CAD build for the part. Positions are in the model's coordinates, mm. A direction names the side the tool comes from. Give positions to 0.01 mm unless a question says otherwise; leave off trailing zeros. Loops run counter-clockwise (first coordinate to the right, second up) from the corner with the lowest first, then second, coordinate; pieces in that order, holes last. Notation, with made-up numbers: M 50,-14 L 100,-14 A18 cw 100,11 Z; hole C 40.25,51 d3. An arc over 180 degrees is marked long. Answer as CSV lines item,"result".
from build123d import *

# Parameters (mm, degrees)
F0_W     = 101.6
F0_H     = 50.8
F1_DEPTH = 6.35
F2_R     = 3.789272
F2_R_2   = 4.108367
F2_R_3   = 4.310253
F2_R_4   = 4.227881
F3_DEPTH = 6.35
F4_W     = 12.7
F4_H     = 31.75
F6_W     = 6.35
F6_H     = 5.291667
F8_SIZE  = 1.27
F9_R     = 1.27
F10_SIZE = 1.27


with BuildPart() as f1:
    # F0 (on Top) → F1 (new body)
    with BuildSketch(Plane.XY):
        Rectangle(F0_W, F0_H)
    extrude(amount=F1_DEPTH)

    # F2 (on face) → F3 (cut)
    with BuildSketch(Plane.XY.offset(6.35)):
        with Locations((-44.241536, 19.306498)):
            Circle(F2_R)
        with Locations((42.667963, 19.790674)):
            Circle(F2_R_2)
        with Locations((43.152139, -17.248752)):
            Circle(F2_R_3)
        with Locations((-44.483624, -17.975016)):
            Circle(F2_R_4)
    extrude(amount=-F3_DEPTH, mode=Mode.SUBTRACT)

    # F4 (on Front) → F5 (revolve)
    with BuildSketch(Plane.XZ):
        with Locations((-6.35, 15.875)):
            Rectangle(F4_W, F4_H)
    revolve(axis=Axis((0, 0, 15.875), (0, 0, 1)))

    # F6 (on Front) → F7 (revolve, cut)
    with BuildSketch(Plane.XZ):
        with Locations((9.708053, 19.931483)):
            Rectangle(F6_W, F6_H)
    revolve(axis=Axis((0, 0, 31.75), (0, 0, -1)), mode=Mode.SUBTRACT)

    # F8
    f8_edges = [f1.edges().sort_by_distance(p)[0] for p in [
        (0, -25.4, 6.35),
        (-50.8, 0, 6.35),
        (0, 25.4, 6.35),
        (50.8, 0, 6.35),
    ]]
    chamfer(f8_edges, length=F8_SIZE)

    # F9
    f9_edges = [f1.edges().sort_by_distance(p)[0] for p in [
        (12.7, 0, 6.35),
        (12.7, 0, 31.75),
    ]]
    fillet(f9_edges, radius=F9_R)

    # F10
    f10_edges = [f1.edges().sort_by_distance(p)[0] for p in [
        (12.7, 0, 17.285649),
    ]]
    chamfer(f10_edges, length=F10_SIZE)


solid = f1.part
1) Mould opens along Y. For faces 1 (the face through (-48.027, 19.473, 3.219)), 2 (the face through (2.75, 12.4, 11.88)), 3 (the face through (6, -3, 22.577)) say: +Y half, -Y half, draft (parallel to the pull), parting line (faces both ways), or undercut.
Answer below:
face 1,"undercut"
face 2,"parting line"
face 3,"draft"
2) Band-saw the part on C-C on z = 20. Give the cut face in (x, y), and give its area (3 significant figures).
Answer below:
outline,"C 0,0 d13.07"
area,"134 mm^2"
3) Band-saw the part on B-B on y = 0. Give the cut face in (x, z).
Answer below:
outline,"M -50.8,0 L 50.8,0 L 50.8,5.08 L 49.53,6.35 L 13.97,6.35 A1.27 cw 12.7,7.62 L 12.7,16.02 L 11.43,17.29 L 6.53,17.29 L 6.53,22.58 L 12.7,22.58 L 12.7,30.48 A1.27 ccw 11.43,31.75 L -11.43,31.75 A1.27 ccw -12.7,30.48 L -12.7,22.58 L -6.53,22.58 L -6.53,17.29 L -11.43,17.29 L -12.7,16.02 L -12.7,7.62 A1.27 cw -13.97,6.35 L -49.53,6.35 L -50.8,5.08 Z"
4) Band-saw the part on A-A on x = 0. Give the cut face in (y, z).
Answer below:
outline,"M -25.4,0 L 25.4,0 L 25.4,5.08 L 24.13,6.35 L 13.97,6.35 A1.27 cw 12.7,7.62 L 12.7,16.02 L 11.43,17.29 L 6.53,17.29 L 6.53,22.58 L 12.7,22.58 L 12.7,30.48 A1.27 ccw 11.43,31.75 L -11.43,31.75 A1.27 ccw -12.7,30.48 L -12.7,22.58 L -6.53,22.58 L -6.53,17.29 L -11.43,17.29 L -12.7,16.02 L -12.7,7.62 A1.27 cw -13.97,6.35 L -24.13,6.35 L -25.4,5.08 Z"
5) Band-saw the part on D-D on x = -33. Give the cut face in (y, z).
Answer below:
outline,"M -25.4,0 L 25.4,0 L 25.4,5.08 L 24.13,6.35 L -24.13,6.35 L -25.4,5.08 Z"
6) Drill centre lines: line 1 (X direction, y = 22.5, z = 4.5); line 2 (Z direction, x = 13.5, y = -16); line 3 (X direction, y = 16.5, z = 2.5). Where is each one in solid material? Low to high. Write a range as from..to.
Answer below:
line 1,"x = -50.8..-46.28, -42.2..39.58, 45.76..50.8"
line 2,"z = 0..6.35"
line 3,"x = -50.8..-46.79, -41.7..40.21, 45.13..50.8"
7) Flat gauge pins, fed straight in: pin 1 (1.5 mm diameter, centred on x = 28.5, y = 6.5, fed in from +Z); pin 2 (6.5 mm diameter, centred on x = 42.67, y = 19.79, fed in from +Z); pin 3 (13.5 mm diameter, centred on x = -44.48, y = -17.98, fed in from -Z); pin 4 (5 mm diameter, centred on y = 6, z = 24.5, fed in from -X). Where does each tip first touch, or does it go through?
Answer below:
pin 1,"stops at z = 6.35"
pin 2,"passes through"
pin 3,"stops at z = 0"
pin 4,"stops at x = -12.21"
8) Which spindle directions (+Z, -Z, +X, -X, +Y, -Y) get a long thin tool onto all of the face, cutting with end or side? Do faces 4 (the face through (-47.6, -15.12, 3.22)), 5 (the face through (2.75, 12.4, 26.58)), 6 (the face through (3.51, -5.51, 19.97)). Say none if no direction does.
Answer below:
face 4,"+Z, -Z"
face 5,"+Z"
face 6,"none"
